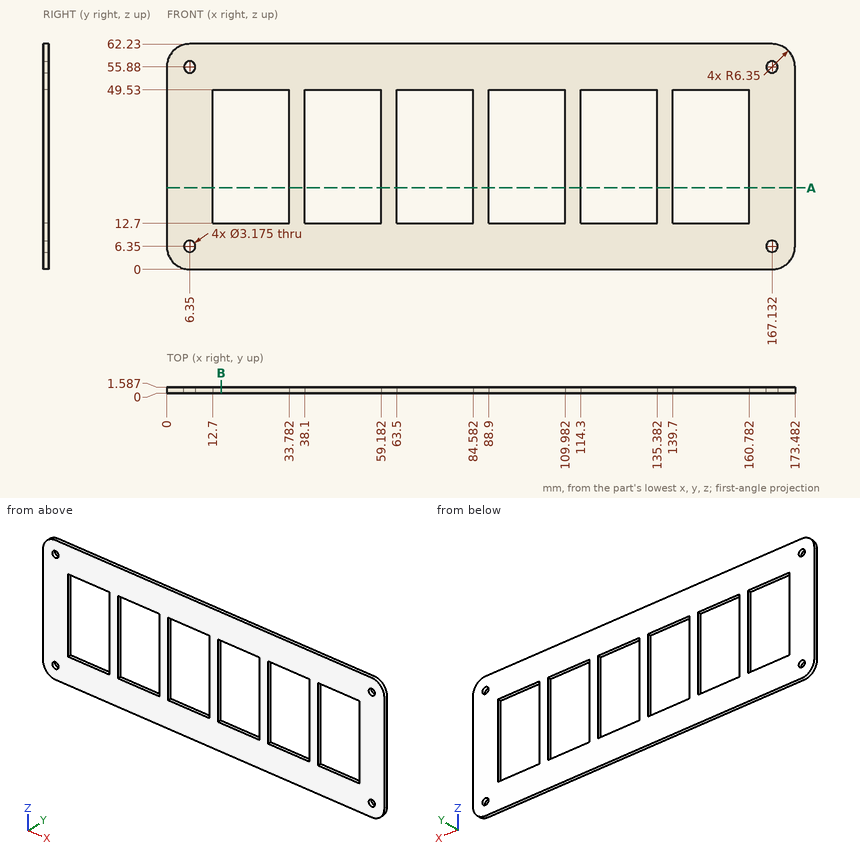
Geometry: see drawing. Coordinates: mm, zero at the bounding-box minimum. Give positions to 0.01 mm unless a question says otherwise; leave off trailing zeros. Loops run counter-clockwise (first coordinate to the right, second up) from the corner with the lowest first, then second, coordinate; pieces in that order, holes last. Notation, with made-up numbers: (-2, 66) - (5, 66) arc R19 cw to (5, 76) - close; hole circle Ø2 at (40, 35.25). An arc over 180 degrees is marked (long way). Use CSV: the item, a comma, the result in double quotes. Start each with the question number.
Item 1: Section A-A on z = 22.5. Return loops of the section in (x, y).
Item 2: Line query: line 1 (Z direction, x = 152.5, y = 1.4); line 2 (X direction, y = 1.5, z = 4). Output: solid intervals per line, ascending.
Item 3: Section B-B on x = 15. Return loops of the section in (y, z).
Item 4: Contact query for flat-ended pins moving along their axis: P1, Ø1.9, axis at x = 167.132, z = 55.88, coming from the -Y side; P2, Ø5, axis at x = 65, z = 14.5, coming from the +Y side. Output: stop coordinate, or through.
Ans:
1,outline,"(0, 0) - (12.7, 0) - (12.7, 1.59) - (0, 1.59) - close; (33.78, 0) - (38.1, 0) - (38.1, 1.59) - (33.78, 1.59) - close; (59.18, 0) - (63.5, 0) - (63.5, 1.59) - (59.18, 1.59) - close; (84.58, 0) - (88.9, 0) - (88.9, 1.59) - (84.58, 1.59) - close; (109.98, 0) - (114.3, 0) - (114.3, 1.59) - (109.98, 1.59) - close; (135.38, 0) - (139.7, 0) - (139.7, 1.59) - (135.38, 1.59) - close; (160.78, 0) - (173.48, 0) - (173.48, 1.59) - (160.78, 1.59) - close"
2,line 1,"z = 0 to 12.7, 49.53 to 62.23"
2,line 2,"x = 0.45 to 173.03"
3,outline,"(0, 0) - (1.59, 0) - (1.59, 12.7) - (0, 12.7) - close; (0, 49.53) - (1.59, 49.53) - (1.59, 62.23) - (0, 62.23) - close"
4,P1,"passes through"
4,P2,"stops at y = 1.59"
